from build123d import *

# Parameters (mm, degrees)
F0_W     = 38
F0_H     = 38
F1_DEPTH = 1
F2_DEPTH = 40
F3_DEPTH = 40
F4_R     = 5


with BuildPart() as f1:
    # F0 (on Top) → F1 (new body)
    with BuildSketch(Plane.XY):
        with Locations((19, 19)):
            Rectangle(F0_W, F0_H)
    extrude(amount=F1_DEPTH)

    # F0 (on Top) → F2 (join)
    with BuildSketch(Plane.XY):
        Polygon((38, 0), (0, 0), (0, 38), (-5, 38), (-5, -5), (43, -5), (43, 38), (38, 38), align=None)
        Polygon((-5, 38), (0, 38), (38, 38), (43, 38), (43, 43), (-5, 43), align=None)
    extrude(amount=F2_DEPTH)

    # F0 (on Top) → F3 (join)
    with BuildSketch(Plane.XY):
        Polygon((-5, 38), (0, 38), (38, 38), (43, 38), (43, 43), (-5, 43), align=None)
    extrude(amount=-F3_DEPTH)

    # F4
    f4_edges = [f1.edges().sort_by_distance(p)[0] for p in [
        (0, 38, 20.5),
        (38, 38, 20.5),
        (38, 0, 20.5),
        (0, 0, 20.5),
    ]]
    fillet(f4_edges, radius=F4_R)


solid = f1.part
Input: part model. Units: mm. Frame: model coordinates. A direction names the side the tool comes from. Coordinates: 2 decimals unless noted, no trailing zeros. Loops run counter-clockwise (first coordinate to the right, second up) from the corner with the lowest first, then second, coordinate; pieces in that order, holes last. Notation, with made-up numbers: (50.25, 50.5) - (90.25, 50.5) arc R37 cw to (90.25, 87.5) - close; hole circle Ø7 at (-33.75, 37.25). An arc over 180 degrees is marked (long way). Answer in a Markdown table with one row per item. Add a question column.
Item 1: Line query: line 1 along X through (y, z) = (6.5, 8.5); line 2 along Z through (x, y) = (6, 26.5). Output: solid intervals per line, ascending. Write a range as [from, to].
Item 2: Section query D-D on y = 36. Return the cut outline in (x, z), then the cut area to 3 significant figures.
Item 3: Access query for faces 1 (the flat face through (43, 19, 18)), 2 (the flat face through (19, 17, 0)), 3 (the flat face through (0, 19, 20)). Directions: +Z, -Z, +X, -X, +Y, -Y. A direction counts if a zero-diameter tool reaches every point of the face in a straight line with its end or side. Return the directions, or none.
Item 4: Contact query for flat-ended pins moving along their axis: P1, Ø4, axis at x = 32.5, z = -21.5, coming from the -Y side; P2, Ø10, axis at x = 24, y = 0.5, coming from the -Z side. Output: stop coordinate, or through.
Item 5: Section query A-A on y = 29. Return the cut outline in (x, z).
Item 6: Mould query, pull axis Y, two halves, no side actions, for faces 4 (the flat face through (19, -5, 20)), 5 (the flat face through (19, 43, 1)), 6 (the flat face through (19, 41, -40)), 7 (the cylindrical face through (37, 2, 21)). Classes: released by +Y, released by -Y, zero draft, split by the parting line, or undercut.
Item 7: Section query C-C on z = 13. Return the cut outline in (x, y).
Item 8: Section query B-B on x = 37. Return the cut outline in (y, z), then the cut area to 3 significant figures.
Recorded:
| question | item | result |
|---|---|---|
| 1 | line 1 | [-5, 0], [38, 43] |
| 1 | line 2 | [0, 1] |
| 2 | outline | (-5, 0) - (43, 0) - (43, 40) - (37, 40) - (37, 1) - (1, 1) - (1, 40) - (-5, 40) - close |
| 2 | area | 516 mm^2 |
| 3 | face 1 | +Z, -Z, +X, +Y, -Y |
| 3 | face 2 | -Z, +X, -X, -Y |
| 3 | face 3 | +Z |
| 4 | P1 | y = 38 |
| 4 | P2 | z = 0 |
| 5 | outline | (-5, 0) - (43, 0) - (43, 40) - (38, 40) - (38, 1) - (0, 1) - (0, 40) - (-5, 40) - close |
| 6 | face 4 | released by -Y |
| 6 | face 5 | released by +Y |
| 6 | face 6 | zero draft |
| 6 | face 7 | undercut |
| 7 | outline | (-5, -5) - (43, -5) - (43, 43) - (-5, 43) - close; hole (0, 5) arc R5 ccw to (5, 0) - (33, 0) arc R5 ccw to (38, 5) - (38, 33) arc R5 ccw to (33, 38) - (5, 38) arc R5 ccw to (0, 33) - close |
| 8 | outline | (-5, 0) - (38, 0) - (38, -40) - (43, -40) - (43, 40) - (36, 40) - (36, 1) - (2, 1) - (2, 40) - (-5, 40) - close |
| 8 | area | 794 mm^2 |
